Input: dimensioned drawing with shaded views. Units: mm. Origin: part minimum x, y, z. Give positions to 0.01 mm unless a question says otherwise; leave off trailing zeros. Write each loop counter-clockwise with the first axis right and the second up, starting at its lowest first coordinate (ties: lowest second). Pieces come first, ordered by that corner, then holes. Notation, with made-up numbers: (59.25, -31.75) -> (83.25, -31.75) arc R21 ccw to (83.25, -2.75) -> close; hole circle Ø10 at (-25, -10.5). An arc over 180 degrees is marked (long way). Answer in a Markdown table with one row per item. Add a question column.
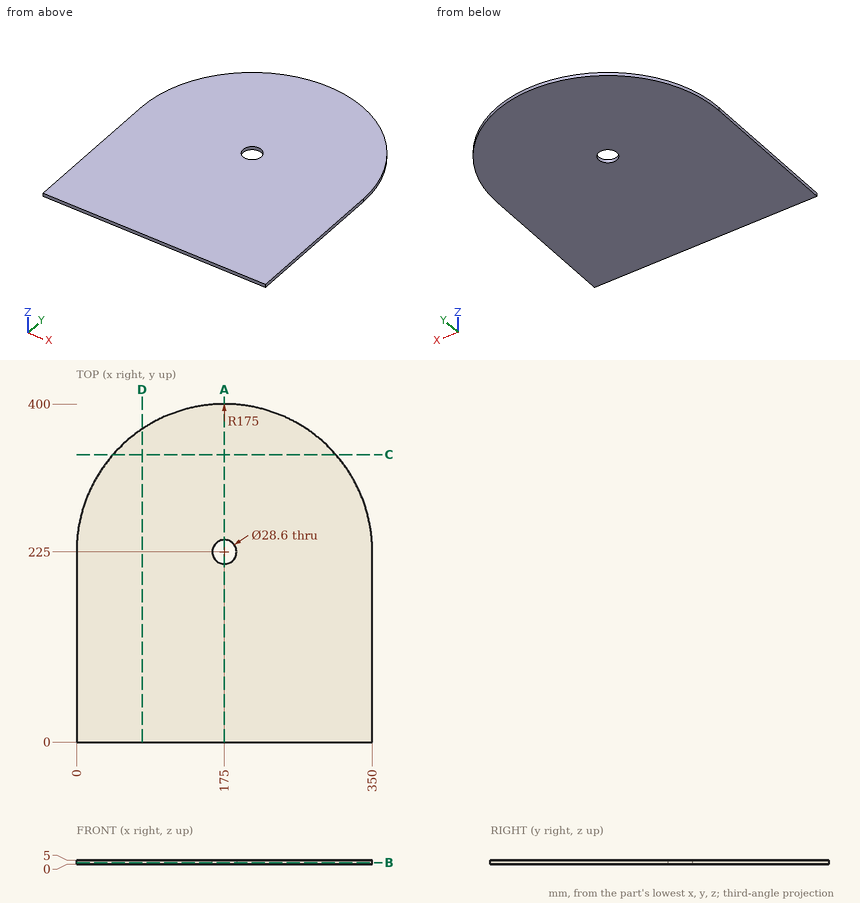
Q1. Section D-D on x = 77.5. Return loops of the section in (y, z), and give its area (3 significant figures).
Q2. Section C-C on y = 340. Return loops of the section in (x, z).
Q3. Section A-A on x = 175. Return loops of the section in (y, z).
Q4. Section B-B on z = 2.1. Return loops of the section in (x, y), and give its area (3 significant figures).
Q5. Line query: probe 1 along Y at (x, z) = (175, 1.6); probe 2 along Y at (x, z) = (186, 1.15); probe 3 along X at (y, z) = (238, 1.25). Output: solid intervals per line, ascending. Write a range as from..to.
Q6. Contact query for a flat-ended pin moving along its axis: pin 1 Ø2 at (x, z) = (261, 3) entering from +Y. Output: stop coordinate, or through.
Checks:
| question | item | result |
|---|---|---|
| 1 | outline | (0, 0) -> (370.32, 0) -> (370.32, 5) -> (0, 5) -> close |
| 1 | area | 1,850 mm^2 |
| 2 | outline | (43.09, 0) -> (306.91, 0) -> (306.91, 5) -> (43.09, 5) -> close |
| 3 | outline | (0, 0) -> (210.7, 0) -> (210.7, 5) -> (0, 5) -> close; (239.3, 0) -> (400, 0) -> (400, 5) -> (239.3, 5) -> close |
| 4 | outline | (0, 0) -> (350, 0) -> (350, 225) arc R175 ccw to (0, 225) -> close; hole circle Ø28.6 at (175, 225) |
| 4 | area | 126,000 mm^2 |
| 5 | probe 1 | 0..210.7, 239.3..400 |
| 5 | probe 2 | 0..215.86, 234.14..399.65 |
| 5 | probe 3 | 0.48..169.04, 180.96..349.52 |
| 6 | pin 1 | y = 377.97 |
